from build123d import *

# Parameters (mm, degrees)
SKETCH1_R           = 20
BOSS_EXTRUDE1_DEPTH = 20
SKETCH2_R           = 30
SKETCH2_R_2         = 20
BOSS_EXTRUDE2_DEPTH = 5


with BuildPart() as part:
    # Sketch1 → Boss-Extrude1 (new body)
    with BuildSketch(Plane(origin=(0, 0, 0), x_dir=(1, 0, 0), z_dir=(0, 1, 0))):
        with BuildLine():
            Line((-100, 140), (-50, 140))
            Line((-50, 140), (-50, 130))
            Line((-50, 130), (-10, 130))
            Line((-10, 130), (-10, 107.320508075))
            ThreePointArc((-10, 107.320508075), (0, 70), (10, 107.320508075))
            Line((10, 107.320508075), (10, 130))
            Line((10, 130), (50, 130))
            Line((50, 130), (50, 140))
            Line((50, 140), (100, 140))
            ThreePointArc((100, 140), (128.284271247, 128.284271247), (140, 100))
            Line((140, 100), (140, 54))
            ThreePointArc((140, 54), (86, 0), (140, -54))
            Line((140, -54), (140, -100))
            ThreePointArc((140, -100), (128.284271247, -128.284271247), (100, -140))
            Line((100, -140), (50, -140))
            Line((50, -140), (50, -130))
            Line((50, -130), (10, -130))
            Line((10, -130), (10, -107.320508076))
            ThreePointArc((10, -107.320508076), (0, -70), (-10, -107.320508076))
            Line((-10, -107.320508076), (-10, -130))
            Line((-10, -130), (-50, -130))
            Line((-50, -130), (-50, -140))
            Line((-50, -140), (-100, -140))
            ThreePointArc((-100, -140), (-128.284271247, -128.284271247), (-140, -100))
            Line((-140, -100), (-140, -54))
            ThreePointArc((-140, -54), (-86, 0), (-140, 54))
            Line((-140, 54), (-140, 100))
            ThreePointArc((-140, 100), (-128.284271247, 128.284271247), (-100, 140))
        make_face()
        with Locations(Location((-100, -100, 0), (0, 0, 270))):
            Circle(SKETCH1_R, mode=Mode.SUBTRACT)
        with Locations(Location((-100, 100, 0), (0, 0, 270))):
            Circle(SKETCH1_R, mode=Mode.SUBTRACT)
        with Locations(Location((100, 100, 0), (0, 0, 90))):
            Circle(SKETCH1_R, mode=Mode.SUBTRACT)
        with Locations(Location((100, -100, 0), (0, 0, 90))):
            Circle(SKETCH1_R, mode=Mode.SUBTRACT)
    extrude(amount=BOSS_EXTRUDE1_DEPTH)

    # Sketch2 → Boss-Extrude2 (add)
    # profile 1 of 4: a face of its own
    with BuildSketch(Plane(origin=(0, 20, 0), x_dir=(1, 0, 0), z_dir=(0, 1, 0))):
        with Locations(Location((-100, 100, 0), (0, 0, 270))):
            Circle(SKETCH2_R)
        with Locations(Location((-100, 100, 0), (0, 0, 270))):
            Circle(SKETCH2_R_2, mode=Mode.SUBTRACT)
    # profile 2 of 4: a face of its own
    with BuildSketch(Plane(origin=(0, 20, 0), x_dir=(1, 0, 0), z_dir=(0, 1, 0))):
        with Locations(Location((100, 100, 0), (0, 0, 90))):
            Circle(SKETCH2_R)
        with Locations(Location((100, 100, 0), (0, 0, 90))):
            Circle(SKETCH2_R_2, mode=Mode.SUBTRACT)
    # profile 3 of 4: a face of its own
    with BuildSketch(Plane(origin=(0, 20, 0), x_dir=(1, 0, 0), z_dir=(0, 1, 0))):
        with Locations(Location((100, -100, 0), (0, 0, 270))):
            Circle(SKETCH2_R)
        with Locations(Location((100, -100, 0), (0, 0, 90))):
            Circle(SKETCH2_R_2, mode=Mode.SUBTRACT)
    # profile 4 of 4: a face of its own
    with BuildSketch(Plane(origin=(0, 20, 0), x_dir=(1, 0, 0), z_dir=(0, 1, 0))):
        with Locations(Location((-100, -100, 0), (0, 0, 90))):
            Circle(SKETCH2_R)
        with Locations(Location((-100, -100, 0), (0, 0, 90))):
            Circle(SKETCH2_R_2, mode=Mode.SUBTRACT)
    extrude(amount=BOSS_EXTRUDE2_DEPTH)


solid = part.part
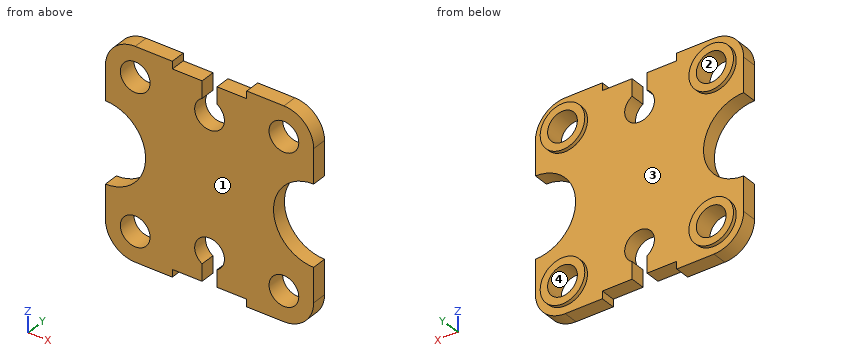
Can you work these out from the model? Positions are in its coordinate system, mm. Face numbers are marked on the shaded views. A direction names the side the tool comes from. Give positions to 0.01 mm unless a question says otherwise; leave off trailing zeros. Loops run counter-clockwise (first coordinate to the right, second up) from the corner with the lowest first, then second, coordinate; pieces in that order, holes last. Notation, with made-up numbers: (45.5, 86) - (102.5, 86) arc R18 ccw to (102.5, 112) - close; hole circle Ø1 at (30.5, 85.25). An arc over 180 degrees is marked (long way). One line per item, written item: value.
(1) I need wall thicknesses on line 1 along X through (y, z) = (9.25, 112); line 2 along Z through (x, y) = (100, 5); line 3 along X through (y, z) = (22.75, 105). Which ranges of each line are inside material? Lowest first, please.
Verdict:
line 1: -138.16 to -116, -84 to -10, 10 to 84, 116 to 138.16
line 2: -140 to -120, -80 to -36.28, 36.28 to 80, 120 to 140
line 3: -129.58 to -119.36, -80.64 to -70.42, 70.42 to 80.64, 119.36 to 129.58
(2) If we mould it in two halves opening along X, with no side actions, what happens to the marked faces 1 and 2? For each: released by +X, released by -X, zero draft, split by the parting line, or undercut.
Verdict:
face 1: zero draft
face 2: undercut
(3) If we section it at B-B, the plane x = -94: List the corners of the cut face in (y, z) for me, plus the area to 3 significant figures.
Verdict:
outline: (0, -140) - (20, -140) - (20, -129.39) - (25, -129.39) - (25, -119.08) - (0, -119.08) - close; (0, -80.92) - (25, -80.92) - (25, -70.61) - (20, -70.61) - (20, -28.28) - (0, -28.28) - close; (0, 28.28) - (20, 28.28) - (20, 70.61) - (25, 70.61) - (25, 80.92) - (0, 80.92) - close; (0, 119.08) - (25, 119.08) - (25, 129.39) - (20, 129.39) - (20, 140) - (0, 140) - close
area: 3,150 mm^2
(4) If we section it at C-C, the plane z = -96: List the corners of the cut face in (x, y) for me, plus the area to 3 significant figures.
Verdict:
outline: (-140, 0) - (-119.6, 0) - (-119.6, 25) - (-129.73, 25) - (-129.73, 20) - (-140, 20) - close; (-80.4, 0) - (-19.08, 0) - (-19.08, 20) - (-70.27, 20) - (-70.27, 25) - (-80.4, 25) - close; (19.08, 0) - (80.4, 0) - (80.4, 25) - (70.27, 25) - (70.27, 20) - (19.08, 20) - close; (119.6, 0) - (140, 0) - (140, 20) - (129.73, 20) - (129.73, 25) - (119.6, 25) - close
area: 3,470 mm^2
(5) I'm going to push flat-ended pins straight in: pin 1 (6 mm diameter, centred on y = 7, z = -116.5, fed in from -X); pin 2 (8 mm diameter, centred on y = 8.5, z = 137.5, fed in from -X); pin 3 (10 mm diameter, centred on x = 29.5, y = 10.5, fed in from -Z). Where does each tip first touch, or does it pass through?
Verdict:
pin 1: x = -137.65
pin 2: x = -121.86
pin 3: z = -130
(6) If we section it at A-A, the plane y = 12.5: State how many separate pieces and enclosed holes the cut face has, plus the area to 3 significant figures.
Verdict:
separate pieces: 1
enclosed holes: 4
area: 57,500 mm^2
(7) On a 3-axis mill with a long thin cutter (end or side, diameter ignored), from which of +Z, -Z, +X, -X, +Y, -Y can I reach the whole of each face in a straight line? I mean the marked faces 3 and 4. Say none if no direction works.
Verdict:
face 3: +Y
face 4: +Y, -Y
(8) If we section it at D-D, the plane x = -58: List the corners of the cut face in (y, z) for me, plus the area to 3 significant figures.
Verdict:
outline: (0, -140) - (20, -140) - (20, 140) - (0, 140) - close
area: 5,600 mm^2
